```python
from build123d import *

# Parameters (mm, degrees)
SKETCH1_R                    = 17.6
BOSS_EXTRUDE1_DEPTH          = 49
F_3_0_3_DIAMETER_HOLE1_D     = 3
F_3_0_3_DIAMETER_HOLE1_DEPTH = 5
F_3_0_3_DIAMETER_HOLE1_TIP   = 0.901290929
SKETCH6_R                    = 2.5
BOSS_EXTRUDE2_DEPTH          = 2
BOSS_EXTRUDE3_START          = 14.5
SKETCH7_R                    = 2.5
BOSS_EXTRUDE3_DEPTH          = 14.5
SKETCH8_R                    = 2
BOSS_EXTRUDE4_DEPTH          = 3
BOSS_EXTRUDE5_START          = 18.5
SKETCH7_2_R                  = 2.5
BOSS_EXTRUDE5_DEPTH          = 1
CHAMFER1_SIZE                = 0.25
CUT_EXTRUDE1_DEPTH           = 57.749625549
CUT_EXTRUDE1_DEPTH_BACK      = 57.749625549
SKETCH9_W                    = 8
SKETCH9_H                    = 0.5


with BuildPart() as part:
    # Sketch1 → Boss-Extrude1 (new body)
    with BuildSketch(Plane(origin=(0, 0, 0), x_dir=(0, 0, -1), z_dir=(1, 0, 0))):
        Circle(SKETCH1_R)
    extrude(amount=BOSS_EXTRUDE1_DEPTH)

    # 3.0 _3_ Diameter Hole1
    with Locations(Plane(origin=(49, 0, 0), x_dir=(0, 0, -1), z_dir=(1, 0, 0))):
        with Locations((0, 12.5), (9.5, 0), (0, -12.5), (-9.5, 0)):
            Hole(F_3_0_3_DIAMETER_HOLE1_D / 2, depth=F_3_0_3_DIAMETER_HOLE1_DEPTH)
            with Locations((0, 0, -(F_3_0_3_DIAMETER_HOLE1_DEPTH + F_3_0_3_DIAMETER_HOLE1_TIP / 2))):  # 118° drill point
                Cone(0, F_3_0_3_DIAMETER_HOLE1_D / 2, F_3_0_3_DIAMETER_HOLE1_TIP, mode=Mode.SUBTRACT)

    # Sketch6 → Boss-Extrude2 (add)
    with BuildSketch(Plane(origin=(49, 0, 0), x_dir=(0, 0, -1), z_dir=(1, 0, 0))):
        Circle(SKETCH6_R)
    extrude(amount=BOSS_EXTRUDE2_DEPTH)

    # Sketch7 → Boss-Extrude3 (add)
    with BuildSketch(Plane.ZY.offset(BOSS_EXTRUDE3_START)):
        with Locations(Location((0, 0, 0), (0, 0, 180))):
            Circle(SKETCH7_R)
    extrude(amount=-BOSS_EXTRUDE3_DEPTH)

    # Sketch8 → Boss-Extrude4 (add)
    with BuildSketch(Plane.ZY.offset(14.5)):
        Circle(SKETCH8_R)
    extrude(amount=BOSS_EXTRUDE4_DEPTH)

    # Sketch7_2 → Boss-Extrude5 (add)
    with BuildSketch(Plane.ZY.offset(BOSS_EXTRUDE5_START)):
        with Locations(Location((0, 0, 0), (0, 0, 180))):
            Circle(SKETCH7_2_R)
    extrude(amount=-BOSS_EXTRUDE5_DEPTH)

    # Chamfer1
    chamfer1_edges = [part.edges().sort_by_distance(p)[0] for p in [
        (0, 0, 17.6),
        (51, 0, 2.5),
        (-18.5, 0, 2.5),
        (49, 0, 17.6),
    ]]
    chamfer(chamfer1_edges, length=CHAMFER1_SIZE)

    # Sketch9 → Cut-Extrude1 (cut, two sides: drawn at the far end of the back side and taken through both)
    with BuildSketch(Plane.XY.offset(-CUT_EXTRUDE1_DEPTH_BACK)):
        with Locations((-6, -2.25)):
            Rectangle(SKETCH9_W, SKETCH9_H)
    extrude(amount=CUT_EXTRUDE1_DEPTH + CUT_EXTRUDE1_DEPTH_BACK, mode=Mode.SUBTRACT)


solid = part.part
```
The listing builds one solid part. Answer for the finished solid, in the listing's coordinates (mm). A direction names the side the tool comes from. Coordinates: 2 decimals unless noted, no trailing zeros. Write each loop counter-clockwise with the first axis right and the second up, starting at its lowest first coordinate (ties: lowest second). Pieces come first, ordered by that corner, then holes. Notation, with made-up numbers: M 52.25,8 L 77.25,8 A15 cw 77.25,18 Z; hole C 34.5,-27.5 d5. An arc over 180 degrees is marked long. Use a Markdown table: item, result. Add a question column.
1. Section B-B (x = 10) is taken. Give the vertices of the cut face in (y, z), plus the area to 3 significant figures.
2. Given P1, Ø6, axis at x = 26.5, z = -4.5, coming from the -Y side; P2, Ø2.5, axis at y = 0, z = 9.5, coming from the +X side; P3, Ø10, axis at x = 4.5, z = 8.5, coming from the -Y side; P4, Ø5, axis at x = -6, z = 6, coming from the +Y side, each flat-ended and moving along its own axis, determine where each tip first touches the part or whether it passes through.
3. Section A-A (x = 47.5) is taken. Give the vertices of the cut face in (y, z).
4. For a pull along X with two mould halves and no side action, classify faces 1 (the flat face through (49, 0, -4)), 2 (the cylindrical face through (46, -14, 0)), 3 (the flat face through (0, 0, -4)), 4 (the flat face through (-6, -2, 0)) as +X half, -X half, draft (parallel to the pull), parting line (faces both ways), or undercut.
5. Straight lines are drawn through the part: line 1 along Y through (x, z) = (47.3, 0); line 2 along X through (y, z) = (-4, -3); line 3 along Y through (x, z) = (45, 9). For each, find the intervals that lie inside material, in ascending order. Write a range as [from, to].
6. Which of the six approach directions +Z, -Z, +X, -X, +Y, -Y give full straight-line access (tool end or side, diameter ignored) to faces 5 (the flat face through (-18.5, 0, 0)), 6 (the flat face through (51, 0, 0)), 7 (the cylindrical face through (-17.9, -0.1, 2.5)), 8 (the cylindrical face through (-16, -2, 0)), 9 (the cylindrical face through (46, 0, 8))?
Data:
| question | item | result |
|---|---|---|
| 1 | outline | C 0,0 d35.2 |
| 1 | area | 973 mm2 |
| 2 | P1 | stops at y = -17.54 |
| 2 | P2 | stops at x = 43.85 |
| 2 | P3 | stops at y = -17.25 |
| 2 | P4 | passes through |
| 3 | outline | C 0,0 d35.2; hole C -12.5,0 d3; hole C 0,-9.5 d3; hole C 0,9.5 d3; hole C 12.5,0 d3 |
| 4 | face 1 | +X half |
| 4 | face 2 | draft |
| 4 | face 3 | -X half |
| 4 | face 4 | undercut |
| 5 | line 1 | y = [-17.6, -14], [-11, 11], [14, 17.6] |
| 5 | line 2 | x = [0, 49] |
| 5 | line 3 | y = [-15.12, -1.41], [1.41, 15.12] |
| 6 | face 5 | +Z, -Z, -X, +Y, -Y |
| 6 | face 6 | +Z, -Z, +X, +Y, -Y |
| 6 | face 7 | -X |
| 6 | face 8 | none |
| 6 | face 9 | +X |
